Design review of the part built by this model. Coordinates are the model's own, in mm. A direction names the side the tool comes from. Coordinates: 2 decimals unless noted, no trailing zeros. Loops run counter-clockwise (first coordinate to the right, second up) from the corner with the lowest first, then second, coordinate; pieces in that order, holes last. Notation, with made-up numbers: M 20,-25.5 L 68,-25.5 A7 ccw 68,-12.5 Z; hole C -2.75,47.25 d1. An arc over 180 degrees is marked long. Answer as a JSON object with one key per item and string values. Group by question number.
1. Consider section C-C (z = -7). State the section outline as (x, y) points, then the cut area to 3 significant figures.
2. Machinability: for faces 5 (the flat face through (19, 6, -3.8)), 6 (the flat face through (0, -4, -6.25)), 7 (the flat face through (-19, -4, -8)), which of the approach directions +Z, -Z, +X, -X, +Y, -Y give a long, thin tool a straight path to every point of the face, cutting with its end or side? Answer none if there is none.
3. Consider section A-A (y = 3). State the section outline as (x, z) points, then the cut area to 3 significant figures.
4. To check wall thickness, follow probe 1 along X at (y, z) = (4.5, 1.75); probe 2 along Z at (x, y) = (-5.5, -1.25); probe 3 along Y at (x, z) = (19.5, 8.25). State the ranges of each line that lie inside material, in increasing order.
5. Insertion check: pin 1 (3 mm diameter, centred on x = -18.5, y = 3, fed in from +Z); pin 2 (1.5 mm diameter, centred on x = -19, z = 4.5, fed in from -Y); pin 3 (2 mm diameter, centred on y = -4, z = -7, fed in from -X); pin 4 (0.5 mm diameter, centred on y = 1, z = -1, fed in from -X). Each pin has a flat end and moves straight along its axis. Give the tip position at first contact, or say it passes through.
6. Consider section B-B (x = 14.5). State the section outline as (y, z) points, then the cut area to 4 significant figures.
7. Consider section D-D (y = -7.5). State the section outline as (x, z) points.
8. Draft analysis for pull direction X (two halves, no side actions). For faces 1 (the flat face through (-14.5, 4, 0)), 2 (the flat face through (-19, -4, 7)), 3 (the flat face through (0, 1.7, 0)), 4 (the flat face through (-19, 4, 3.75)), state which applies: +X half, -X half, draft (parallel to the pull), parting line (faces both ways), or undercut.
from build123d import *

# Parameters (mm, degrees)
SKETCH_1_W      = 43
SKETCH_1_H      = 17.5
EXTRUDE_1_DEPTH = 1.7
SKETCH_2_W      = 5
SKETCH_2_H      = 3.8
EXTRUDE_2_DEPTH = 8.5
SKETCH_2_3_W    = 7
SKETCH_2_3_H    = 3.75
EXTRUDE_3_DEPTH = 4
SKETCH_4_W      = 38
SKETCH_4_H      = 2.5
EXTRUDE_4_DEPTH = 8.5


with BuildPart() as part:
    # Sketch 1 → Extrude 1 (new body)
    with BuildSketch(Plane(origin=(0, 0, 0), x_dir=(1, 0, 0), z_dir=(0, 1, 0))):
        Rectangle(SKETCH_1_W, SKETCH_1_H)
    extrude(amount=EXTRUDE_1_DEPTH)

    # Sketch 2 → Extrude 2 (add)
    with BuildSketch(Plane(origin=(0, 1.7, 0), x_dir=(1, 0, 0), z_dir=(0, 1, 0))):
        with Locations((19, -1.9)):
            Rectangle(SKETCH_2_W, SKETCH_2_H)
        with Locations((19, 1.9)):
            Rectangle(SKETCH_2_W, SKETCH_2_H)
    extrude(amount=EXTRUDE_2_DEPTH)

    # Sketch 2_3 → Extrude 3 (add)
    with BuildSketch(Plane(origin=(0, 1.7, 0), x_dir=(1, 0, 0), z_dir=(0, 1, 0))):
        with Locations((-18, 1.875)):
            Rectangle(SKETCH_2_3_W, SKETCH_2_3_H)
        with Locations((-18, -1.875)):
            Rectangle(SKETCH_2_3_W, SKETCH_2_3_H)
        Polygon((-21.5, -3.75), (-21.5, 0), (-21.5, 3.75), (-23.8, 3.75), (-23.8, -3.75), align=None)
    extrude(amount=EXTRUDE_3_DEPTH)

    # Sketch 4 → Extrude 4 (add)
    with BuildSketch(Plane.XZ):
        with Locations((0, 7.5)):
            Rectangle(SKETCH_4_W, SKETCH_4_H)
        with Locations((0, -7.5)):
            Rectangle(SKETCH_4_W, SKETCH_4_H)
    extrude(amount=EXTRUDE_4_DEPTH)


solid = part.part
Findings below:
{
 "1": {"outline": "M -21.5,0 L -19,0 L -19,-8.5 L 19,-8.5 L 19,0 L 21.5,0 L 21.5,1.7 L -21.5,1.7 Z", "area": "396 mm^2"},
 "2": {"face 5": "-Z, +X, -X, +Y", "face 6": "+X, -X, -Y", "face 7": "+Z, -Z, -X, -Y"},
 "3": {"outline": "M -23.8,-3.75 L -14.5,-3.75 L -14.5,3.75 L -23.8,3.75 Z; M 16.5,-3.8 L 21.5,-3.8 L 21.5,3.8 L 16.5,3.8 Z", "area": "108 mm^2"},
 "4": {"probe 1": "x = -23.8 to -14.5, 16.5 to 21.5", "probe 2": "z = -8.75 to -6.25, 6.25 to 8.75", "probe 3": "y = 0 to 1.7"},
 "5": {"pin 1": "stops at z = 8.75", "pin 2": "stops at y = 0", "pin 3": "stops at x = -19", "pin 4": "stops at x = -21.5"},
 "6": {"outline": "M -8.5,-8.75 L 1.7,-8.75 L 1.7,8.75 L -8.5,8.75 L -8.5,6.25 L 0,6.25 L 0,-6.25 L -8.5,-6.25 Z", "area": "72.25 mm^2"},
 "7": {"outline": "M -19,-8.75 L 19,-8.75 L 19,-6.25 L -19,-6.25 Z; M -19,6.25 L 19,6.25 L 19,8.75 L -19,8.75 Z"},
 "8": {"face 1": "undercut", "face 2": "-X half", "face 3": "undercut", "face 4": "draft"}
}
